Verification items for the finished model (mm, model axes). A direction names the side the tool comes from. Give positions to 0.01 mm unless a question says otherwise; leave off trailing zeros. Order: outer loops, then holes, each group sorted by start corner. A loop starts at its lowest first (then second) coordinate and runs counter-clockwise, first axis right, second up.
from build123d import *

# Parameters (mm, degrees)
BOSS_EXTRU_1_DEPTH      = 2
BOSS_EXTRU_1_DEPTH_BACK = 21
ESQUISSE1_W             = 21
ESQUISSE1_H             = 80
ESQUISSE10_W            = 3
ESQUISSE10_H            = 80
BOSS_EXTRU_2_DEPTH      = 24.2
ESQUISSE11_W            = 34
ESQUISSE11_H            = 15
ENL_V_MAT_EXTRU_1_DEPTH = 3
CONG_1_R                = 5
ENL_V_MAT_EXTRU_2_DEPTH = 81
COQUE2_START            = -21
COQUE2_OUTLINE_W        = 17
COQUE2_OUTLINE_H        = 76
COQUE2_DEPTH            = 21
ESQUISSE15_W            = 16
ESQUISSE15_H            = 10
ENL_V_MAT_EXTRU_3_DEPTH = 2
ESQUISSE12_R            = 5
ENL_V_MAT_EXTRU_4_DEPTH = 0.7


# Read off the part's stored shape, not the designer's step: Coque2
with BuildPart() as part:
    # Esquisse1 → Boss.-Extru.1 (new, two sides: drawn at the far end of the back side and taken through both)
    with BuildSketch(Plane(origin=(0, 0, 0), x_dir=(1, 0, 0), z_dir=(0, 1, 0)).offset(-BOSS_EXTRU_1_DEPTH_BACK)):
        with Locations((-10.5, -40)):
            Rectangle(ESQUISSE1_W, ESQUISSE1_H)
    extrude(amount=BOSS_EXTRU_1_DEPTH + BOSS_EXTRU_1_DEPTH_BACK)

    # Esquisse10 → Boss.-Extru.2 (add)
    with BuildSketch(Plane(origin=(0, 2, 0), x_dir=(1, 0, 0), z_dir=(0, 1, 0))):
        with Locations((-10.5, -40)):
            Rectangle(ESQUISSE10_W, ESQUISSE10_H)
    extrude(amount=BOSS_EXTRU_2_DEPTH)

    # Esquisse11 → Enlèv. mat.-Extru.1 (cut)
    with BuildSketch(Plane.ZY.offset(12)):
        with Locations((40, 9.5)):
            Rectangle(ESQUISSE11_W, ESQUISSE11_H)
    extrude(amount=-ENL_V_MAT_EXTRU_1_DEPTH, mode=Mode.SUBTRACT)

    # Congé1
    cong_1_edges = [part.edges().sort_by_distance(p)[0] for p in [
        (-10.5, 17, 57),
        (-10.5, 2, 57),
        (-10.5, 2, 23),
        (-10.5, 17, 23),
    ]]
    fillet(cong_1_edges, radius=CONG_1_R)

    # Esquisse13 → Enlèv. mat.-Extru.2 (cut)
    with BuildSketch(Plane.XY.offset(80)):
        Polygon((-12, 26.2), (-9, 26.2), (-9, 24.3), align=None)
    extrude(amount=-ENL_V_MAT_EXTRU_2_DEPTH, mode=Mode.SUBTRACT)

    # Coque2 outline → Coque2 (cut)
    with BuildSketch(Plane(origin=(0, 0, 0), x_dir=(1, 0, 0), z_dir=(0, 1, 0)).offset(COQUE2_START)):
        with Locations((-10.5, -40)):
            Rectangle(COQUE2_OUTLINE_W, COQUE2_OUTLINE_H)
    extrude(amount=COQUE2_DEPTH, mode=Mode.SUBTRACT)

    # Esquisse15 → Enlèv. mat.-Extru.3 (cut)
    with BuildSketch(Plane.ZY.offset(21)):
        with Locations((40, -16)):
            Rectangle(ESQUISSE15_W, ESQUISSE15_H)
    extrude(amount=-ENL_V_MAT_EXTRU_3_DEPTH, mode=Mode.SUBTRACT)

    # Esquisse12 → Enlèv. mat.-Extru.4 (cut)
    with BuildSketch(Plane(origin=(-9, 0, 0), x_dir=(0, 0, -1), z_dir=(1, 0, 0))):
        with Locations((-69.5, 8)):
            Circle(ESQUISSE12_R)
        with Locations((-10.5, 8)):
            Circle(ESQUISSE12_R)
    extrude(amount=-ENL_V_MAT_EXTRU_4_DEPTH, mode=Mode.SUBTRACT)


solid = part.part
(1) Release check for a two-part mould opening along X. For faces 1 (the flat face through (-11, -8, 80)), 2 (the flat face through (-11, -11, 78)), 3 (the flat face through (0, -10, 41)) record: pulls with the +X half, pulls with the -X half, needs draft (parallel to the pull), parting line crosses it, or undercut.
Solved:
face 1: needs draft
face 2: undercut
face 3: pulls with the +X half
(2) Section check B-B, the plane z = 69.5. Enter the section's corners in (x, y).
Solved:
outline: (-21, -21) - (-19, -21) - (-19, 0) - (-2, 0) - (-2, -21) - (0, -21) - (0, 2) - (-9, 2) - (-9, 3) - (-9.7, 3) - (-9.7, 13) - (-9, 13) - (-9, 24.3) - (-12, 26.2) - (-12, 2) - (-21, 2) - close
(3) Go/stop test with flat-tipped pins: pin 1 (9 mm diameter, centred on y = 8, z = 69.5, fed in from -X); pin 2 (5 mm diameter, centred on y = 8, z = 12.5, fed in from +X); pin 3 (2.5 mm diameter, centred on x = -11, z = 38.5, fed in from -Y); pin 4 (4 mm diameter, centred on x = -6, y = 5.5, fed in from -Z). Record where each tip stops, or that it passes through.
Solved:
pin 1: stops at x = -12
pin 2: stops at x = -9.7
pin 3: stops at y = 0
pin 4: passes through
(4) Set-up check for faces 4 (the cylindrical face through (-9.345, 6.085, 64.881)), 5 (the flat face through (-11, -11, 2)), 6 (the flat face through (-11, 9, 23)): record each of +Z, -Z, +X, -X, +Y, -Y from which the full face is reachable in a straight line by a thin tool's end or side.
Solved:
face 4: +X
face 5: -Y
face 6: +X, -X
(5) Section check D-D, the plane z = 29.5. Enter the section's corners in (x, y).
Solved:
outline: (-21, -21) - (-19, -21) - (-19, 0) - (-2, 0) - (-2, -21) - (0, -21) - (0, 2) - (-21, 2) - close; (-12, 17) - (-9, 17) - (-9, 24.3) - (-12, 26.2) - close
(6) Scan lines: line 1 (X direction, y = -2, z = 12); line 2 (Z direction, x = -3.25, y = -14); line 3 (X direction, y = -12.5, z = 42.5). Record each from-to range of solid material in increasing order.
Solved:
line 1: x = -21 to -19, -2 to 0
line 2: z = 0 to 2, 78 to 80
line 3: x = -2 to 0
(7) Section check A-A, the plane y = 8. Enter the section's corners in (x, z), then the cut area to 3 significant figures.
Solved:
outline: (-12, 0) - (-9, 0) - (-9, 5.5) - (-9.7, 5.5) - (-9.7, 15.5) - (-9, 15.5) - (-9, 23) - (-12, 23) - close; (-12, 57) - (-9, 57) - (-9, 64.5) - (-9.7, 64.5) - (-9.7, 74.5) - (-9, 74.5) - (-9, 80) - (-12, 80) - close
area: 124 mm2
(8) Section check C-C, the plane x = -7. Enter the section's corners in (y, z), then the cut area to 3 significant figures.
Solved:
outline: (-21, 0) - (2, 0) - (2, 80) - (-21, 80) - (-21, 78) - (0, 78) - (0, 2) - (-21, 2) - close
area: 244 mm2
